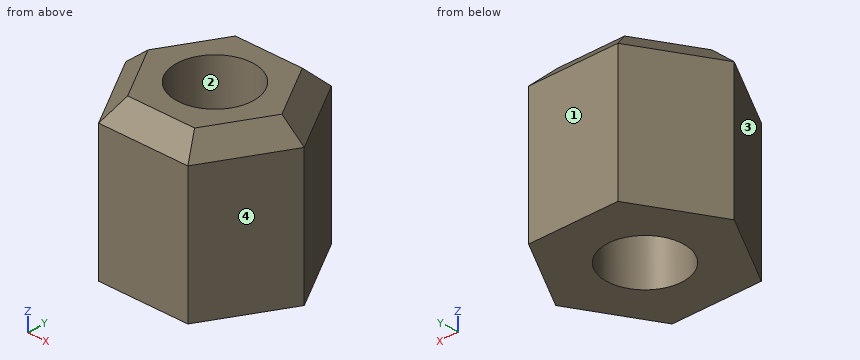
Autodesk Inventor part; units mm, degrees
ref_plane "YZ Plane" through (0, 0, 0) normal (1, 0, 0) x (0, 1, 0)
ref_plane "XZ Plane" through (0, 0, 0) normal (0, 1, 0) x (-1, 0, 0)
ref_plane "XY Plane" through (0, 0, 0) normal (0, 0, 1) x (1, 0, 0)
sketch "Sketch1" plane through (0, 0, 0) normal (0, 0, 1) x (1, 0, 0)
  line L0 (7.3323, 0) -> (3.6662, -6.35)
  line L1 (3.6662, -6.35) -> (-3.6662, -6.35)
  line L2 (-3.6662, -6.35) -> (-7.3323, 0)
  line L3 (-7.3323, 0) -> (-3.6662, 6.35)
  line L4 (-3.6662, 6.35) -> (3.6662, 6.35)
  line L5 (3.6662, 6.35) -> (7.3323, 0)
  point P0 (0, 0)
  point P1 (0, 0)
  dimension "d0" = 12.7
extrude "Extrusion1" add sketch "Sketch1" along normal blind 12.7
sketch "Sketch2" plane through (0, 0, 12.7) normal (0, 0, 1) x (1, 0, 0)
  circle A0 centre (0, 0) radius 3.175
  dimension "d3" = 6.35
extrude "Extrusion2" cut sketch "Sketch2" against normal blind 12.7
chamfer "Chamfer1" distance 1.5875 angle 45 6 edges at (5.4993, 3.175, 12.7) (0, 6.35, 12.7) (-5.4993, 3.175, 12.7) (-5.4993, -3.175, 12.7) (0, -6.35, 12.7) (5.4993, -3.175, 12.7)
properties part number "Bevel Hex Shaft V2"
Can you work these out from the model? Positions are in its coordinate system, mm. Face numbers are marked on the shaded views. Give positions to 0.01 mm unless a question says otherwise; leave off trailing zeros. Loops run counter-clockwise (first coordinate to the right, second up) from the corner with the lowest first, then second, coordinate; pieces in that order, holes last. Notation, with made-up numbers: (52.5, 12.5) - (79.5, 12.5) arc R21 cw to (79.5, 42.5) - close; hole circle Ø10 at (11, 78). An arc over 180 degrees is marked (long way). Answer as a JSON object with one key per item and string values.
Q1. If we mould it in two halves opening along X, with no side actions, what happens to the marked faces 1, 2, 3 and 4? For each: pulls with the +X half, pulls with the -X half, needs draft (parallel to the pull), parting line crosses it, or undercut.
Geometry says:
{"face 1": "needs draft", "face 2": "undercut", "face 3": "pulls with the -X half", "face 4": "pulls with the +X half"}
Q2. Imagine slicing it at D-D on x = -5. Write out the boundary of the cut face in (y, z).
Geometry says:
{"outline": "(-4.04, 0) - (4.04, 0) - (4.04, 11.11) - (0.86, 12.7) - (-0.86, 12.7) - (-4.04, 11.11) - close"}
Q3. Imagine slicing it at A-A on z = 2.75. Write out the boundary of the cut face in (x, y) (3 decimals), plus the area to 3 significant figures.
Geometry says:
{"outline": "(-7.332, 0) - (-3.666, -6.35) - (3.666, -6.35) - (7.332, 0) - (3.666, 6.35) - (-3.666, 6.35) - close; hole circle Ø6.35 at (0, 0)", "area": "108 mm²"}
Q4. Will these pins go through, and if not, where does the flat tip stop? P1, Ø1, axis at y = 4.5, z = 8, coming from the +X side; P2, Ø1.5, axis at y = 1.5, z = 6, coming from the -X side; P3, Ø3, axis at x = -5.5, y = 0.5, coming from the -Z side; P4, Ø5, axis at x = 0, y = 0, coming from the +Z side.
Geometry says:
{"P1": "x = 5.02", "P2": "x = -6.9", "P3": "z = 0", "P4": "through"}
Q5. If I drill on L1, parallel to Y at x = 0, z = 6.5 (3 decimals); L2, parallel to Y at x = -1, z = 6.5; L3, parallel to X at y = 2.25, z = 9, over which ranges is the centre line in solid material (lowest first)?
Geometry says:
{"L1": "-6.35 to -3.175, 3.175 to 6.35", "L2": "-6.35 to -3.01, 3.01 to 6.35", "L3": "-6.03 to -2.24, 2.24 to 6.03"}
Q6. Imagine slicing it at C-C on y = -2.25. Write out the boundary of the cut face in (x, z).
Geometry says:
{"outline": "(-6.03, 0) - (-2.24, 0) - (-2.24, 12.7) - (-4.2, 12.7) - (-6.03, 11.11) - close; (2.24, 0) - (6.03, 0) - (6.03, 11.11) - (4.2, 12.7) - (2.24, 12.7) - close"}
